Can you work these out from the model? Positions are in its coordinate system, mm. A direction names the side the tool comes from. Round coordinates to 2 decimals unless told otherwise and drop trailing zeros. Loops run counter-clockwise (first coordinate to the right, second up) from the corner with the lowest first, then second, coordinate; pieces in that order, holes last. Notation, with made-up numbers: (80.5, -31) -> (105.5, -31) arc R19 cw to (105.5, -4) -> close; hole circle Ø9 at (23.5, 31). An arc over 180 degrees is marked (long way). Write item = value, one per line.
from build123d import *

# Parameters (mm, degrees)
SKETCH_1_W          = 81
SKETCH_1_H          = 86.3
EXTRUDE_1_DEPTH     = 2
SKETCH_2_R          = 1.2
CUT_EXTRUDE_1_DEPTH = 2
SKETCH_3_W          = 2
SKETCH_3_H          = 5
EXTRUDE_2_DEPTH     = 0.8
SKETCH_4_W          = 4
SKETCH_4_H          = 5
EXTRUDE_3_DEPTH     = 2


with BuildPart() as part:
    # ｽｹｯﾁ1 → ﾎﾞｽ - 押し出し1 (new body)
    with BuildSketch(Plane(origin=(0, 0, 0), x_dir=(1, 0, 0), z_dir=(0, 1, 0))):
        Rectangle(SKETCH_1_W, SKETCH_1_H)
    extrude(amount=EXTRUDE_1_DEPTH)

    # ｽｹｯﾁ2 → ｶｯﾄ - 押し出し1 (cut)
    with BuildSketch(Plane(origin=(0, 2, 0), x_dir=(1, 0, 0), z_dir=(0, 1, 0))):
        with Locations(Location((-34, -38.15, 0), (0, 0, 270))):
            Circle(SKETCH_2_R)
        with Locations(Location((-34, 38.15, 0), (0, 0, 270))):
            Circle(SKETCH_2_R)
        with Locations(Location((34, 38.15, 0), (0, 0, 270))):
            Circle(SKETCH_2_R)
        with Locations(Location((34, -38.15, 0), (0, 0, 270))):
            Circle(SKETCH_2_R)
        with Locations(Location((-24.55, 13.3, 0), (0, 0, 270))):
            Circle(SKETCH_2_R)
        with Locations(Location((24.55, 13.3, 0), (0, 0, 270))):
            Circle(SKETCH_2_R)
        with Locations(Location((-11.5, 33.15, 0), (0, 0, 270))):
            Circle(SKETCH_2_R)
        with Locations(Location((11.5, 33.15, 0), (0, 0, 270))):
            Circle(SKETCH_2_R)
        with Locations(Location((-4, 13.3, 0), (0, 0, 270))):
            Circle(SKETCH_2_R)
        with Locations(Location((4, 13.3, 0), (0, 0, 270))):
            Circle(SKETCH_2_R)
    extrude(amount=-CUT_EXTRUDE_1_DEPTH, mode=Mode.SUBTRACT)

    # ｽｹｯﾁ3 → ﾎﾞｽ - 押し出し2 (add)
    with BuildSketch(Plane.XZ):
        with Locations((-39.5, -40.65)):
            Rectangle(SKETCH_3_W, SKETCH_3_H)
        with Locations((39.5, -40.65)):
            Rectangle(SKETCH_3_W, SKETCH_3_H)
    extrude(amount=EXTRUDE_2_DEPTH)

    # ｽｹｯﾁ4 → ﾎﾞｽ - 押し出し3 (add)
    with BuildSketch(Plane.XZ.offset(0.8)):
        with Locations((-40.5, -40.65)):
            Rectangle(SKETCH_4_W, SKETCH_4_H)
        with Locations((40.5, -40.65)):
            Rectangle(SKETCH_4_W, SKETCH_4_H)
    extrude(amount=EXTRUDE_3_DEPTH)


solid = part.part
1. Suppose I cut it at D-D, the plane x = 34. List the corners of the cut face in (y, z) for me.
Entries:
outline = (0, -43.15) -> (2, -43.15) -> (2, -39.35) -> (0, -39.35) -> close; (0, -36.95) -> (2, -36.95) -> (2, 36.95) -> (0, 36.95) -> close; (0, 39.35) -> (2, 39.35) -> (2, 43.15) -> (0, 43.15) -> close
2. I need wall thicknesses on line 1 (X direction, y = 1.2, z = -38.15); line 2 (X direction, y = 1.35, z = -13.3); line 3 (X direction, y = 0.2, z = 26). Which ranges of each line are inside material? Lowest first, please. Write a range as [from, to].
Entries:
line_1 = [-40.5, -35.2], [-32.8, 32.8], [35.2, 40.5]
line_2 = [-40.5, -25.75], [-23.35, -5.2], [-2.8, 2.8], [5.2, 23.35], [25.75, 40.5]
line_3 = [-40.5, 40.5]
3. Suppose I cut it at C-C, the plane z = 38.15. List the corners of the cut face in (x, y) for me.
Entries:
outline = (-40.5, 0) -> (-35.2, 0) -> (-35.2, 2) -> (-40.5, 2) -> close; (-32.8, 0) -> (32.8, 0) -> (32.8, 2) -> (-32.8, 2) -> close; (35.2, 0) -> (40.5, 0) -> (40.5, 2) -> (35.2, 2) -> close
4. Suppose I cut it at A-A, the plane z = -13.3. List the corners of the cut face in (x, y) for me, and give its area (3 significant figures).
Entries:
outline = (-40.5, 0) -> (-25.75, 0) -> (-25.75, 2) -> (-40.5, 2) -> close; (-23.35, 0) -> (-5.2, 0) -> (-5.2, 2) -> (-23.35, 2) -> close; (-2.8, 0) -> (2.8, 0) -> (2.8, 2) -> (-2.8, 2) -> close; (5.2, 0) -> (23.35, 0) -> (23.35, 2) -> (5.2, 2) -> close; (25.75, 0) -> (40.5, 0) -> (40.5, 2) -> (25.75, 2) -> close
area = 143 mm²
5. For faces 4 (the cylindrical face through (10.33, 1.01, -33.41)), 5 (the flat face through (38.5, -1, -41)), 6 (the flat face through (-42, -0.8, -41)), 7 (the flat face through (41, -0.8, -41)), which set-ups out of +Z, -Z, +X, -X, +Y, -Y let a thin tool reach every point of the face, with its end or its side?
Entries:
face_4 = +Y, -Y
face_5 = +Z, -Z, -Y
face_6 = +Z, -Z, -X, +Y
face_7 = +Z, -Z, +X, +Y
6. Suppose I cut it at B-B, the plane x = 4. List the corners of the cut face in (y, z) for me, and give its area (3 significant figures).
Entries:
outline = (0, -43.15) -> (2, -43.15) -> (2, -14.5) -> (0, -14.5) -> close; (0, -12.1) -> (2, -12.1) -> (2, 43.15) -> (0, 43.15) -> close
area = 168 mm²
7. We'd pull the mould along Z, two halves only. Please class faces 1 (the flat face through (-1, 1, 43.15)), 2 (the flat face through (-40.5, 1, -1)), 3 (the cylindrical face through (23.38, 1.01, -13.56)): released by +Z, released by -Z, zero draft, split by the parting line, or undercut.
Entries:
face_1 = released by +Z
face_2 = zero draft
face_3 = undercut
8. I'm going to push flat-ended pins straight in: pin 1 (8 mm diameter, centred on x = 20.5, z = -12, fed in from -Y); pin 2 (2 mm diameter, centred on y = 0, z = -13.5, fed in from -X); pin 3 (1.4 mm diameter, centred on x = 11.5, z = -33.15, fed in from +Y); pin 4 (0.8 mm diameter, centred on x = -41, y = -2, fed in from +Z). Where does each tip first touch, or does it pass through?
Entries:
pin_1 = 0
pin_2 = -40.5
pin_3 = through
pin_4 = -38.15
